Autodesk Inventor part; units mm, degrees
ref_plane "YZ Plane" through (0, 0, 0) normal (1, 0, 0) x (0, 1, 0)
ref_plane "XZ Plane" through (0, 0, 0) normal (0, 1, 0) x (-1, 0, 0)
ref_plane "XY Plane" through (0, 0, 0) normal (0, 0, 1) x (1, 0, 0)
sketch "Sketch1" plane through (0, 0, 0) normal (0, 1, 0) x (-1, 0, 0)
  line L0 (-37.5, 55) -> (37.5, 55)
  line L1 (37.5, 55) -> (37.5, -55)
  line L2 (37.5, -55) -> (-37.5, -55)
  line L3 (-37.5, -55) -> (-37.5, 55)
  line L4 (-37.5, 55) -> (37.5, -55) construction
  line L5 (37.5, 55) -> (-37.5, -55) construction
  point P0 (0, 0)
  dimension "d0" = 75
  dimension "d1" = 110
extrude "Extrusion1" add sketch "Sketch1" along normal blind 5
sketch "Sketch2" plane through (0, 5, 0) normal (0, 1, 0) x (1, 0, 0)
  line L0 (37.5, -55) -> (37.5, 55)
  line L1 (-37.5, -55) -> (37.5, -55)
  line L2 (37.5, 55) -> (-37.5, 55)
  line L3 (-37.5, 55) -> (-37.5, -55)
  point P0 (0, 0)
  point P1 (32.5, -50)
  point P2 (32.5, 50)
  point P3 (-32.5, 50)
  point P4 (-32.5, -50)
  dimension "HS" = 5
  dimension "d12" = 5
  dimension "d13" = 5
  dimension "d14" = 5
hole "Hole1" at (32.5, 5, 50) at (32.5, 5, -50) at (-32.5, 5, -50) at (-32.5, 5, 50) direction (0, -1, 0) diameter 3.2 depth 6
properties part number "DAQ_HousingCover_V1"
Could you check a few things on this model? Use its own coordinates, in mm. Coordinates: 2 decimals unless noted, no trailing zeros. Order: outer loops, then holes, each group sorted by start corner. A loop starts at its lowest first (then second) coordinate and runs counter-clockwise, first axis right, second up. Notation, with made-up numbers: (31.25, 26) - (73.25, 26) arc R25 cw to (73.25, 52) - close; hole circle Ø8 at (33.25, 55.5). An arc over 180 degrees is marked (long way). Answer in a Markdown table with one row per item. Add a question column.
(1) I need wall thicknesses on L1, parallel to Z at x = -32.5, y = 3.35; L2, parallel to X at y = 1, z = -50. Which ranges of each line are inside material? Lowest first, please.
(2) If we section it at B-B, the plane z = -50: Please give me the cut outline in (x, y).
(3) If we section it at A-A, the plane x = 32.5: Please give me the cut outline in (y, z), then the cut area to 3 significant figures.
(4) If we mould it in two halves opening along Z, with no side actions, what happens to faces 1 (the face through (-31.08, 2.46, -49.26)), 2 (the face through (1, 2, 55)), 3 (the face through (33.92, 2.46, -49.26)), 4 (the face through (1, 5, 1))? For each: released by +Z, released by -Z, zero draft, split by the parting line, or undercut.
Results are:
| question | item | result |
|---|---|---|
| 1 | L1 | z = -55 to -51.6, -48.4 to 48.4, 51.6 to 55 |
| 1 | L2 | x = -37.5 to -34.1, -30.9 to 30.9, 34.1 to 37.5 |
| 2 | outline | (-37.5, 0) - (-34.1, 0) - (-34.1, 5) - (-37.5, 5) - close; (-30.9, 0) - (30.9, 0) - (30.9, 5) - (-30.9, 5) - close; (34.1, 0) - (37.5, 0) - (37.5, 5) - (34.1, 5) - close |
| 3 | outline | (0, -55) - (5, -55) - (5, -51.6) - (0, -51.6) - close; (0, -48.4) - (5, -48.4) - (5, 48.4) - (0, 48.4) - close; (0, 51.6) - (5, 51.6) - (5, 55) - (0, 55) - close |
| 3 | area | 518 mm2 |
| 4 | face 1 | undercut |
| 4 | face 2 | released by +Z |
| 4 | face 3 | undercut |
| 4 | face 4 | zero draft |
